Geometry: final body of the model. Coordinates: model frame, mm. Face numbers are marked on the shaded views. Give positions to 0.01 mm unless a question says otherwise; leave off trailing zeros. Loops run counter-clockwise (first coordinate to the right, second up) from the corner with the lowest first, then second, coordinate; pieces in that order, holes last.
1. Section B-B, the plane z = 1.15. Output: boundary loops of the cut face in (x, y).
2. Draft query along Y for the marked faces 1, 2 and 3. Return one class per face: +Y half, -Y half, draft (parallel to the pull), parting line (faces both ways), or undercut.
3. Section A-A, the plane y = 0. Output: boundary loops of the cut face in (x, z), then the cut area to 3 significant figures.
4. Material intervals for line 1 along Y through (x, z) = (0, 1.5); line 2 along Y through (x, z) = (-3.5, 2.55); line 3 along X through (y, z) = (-15.5, 2.9), sorted ascending.
5. First-contact query: P1, Ø1, axis at y = -17.5, z = 1, coming from the +X side; P2, Ø13, axis at x = 0, y = 0, coming from the +Z side; P3, Ø4, axis at x = 27, y = -12, coming from the +Z side; P4, Ø5.5, axis at x = 0, y = 14, coming from the +Z side. Flat tips, straight axial feed; report the tip coordinate or a pass-through.
6. Section C-C, the plane x = 14. Output: boundary loops of the cut face in (y, z).
from build123d import *

# Parameters (mm, degrees)
SKETCH1_R                                           = 36.8
BOSS_EXTRUDE1_DEPTH                                 = 5
CUT_EXTRUDE1_REACH                                  = 54.283
SKETCH2_R                                           = 4
CUT_EXTRUDE2_DEPTH                                  = 2
CUT_EXTRUDE3_DEPTH                                  = 2
CSK_FOR_M3_FLAT_COUNTERSUNK_HEAD_SCREW1_D           = 3.4
CSK_FOR_M3_FLAT_COUNTERSUNK_HEAD_SCREW1_DEPTH       = 9
CSK_FOR_M3_FLAT_COUNTERSUNK_HEAD_SCREW1_CSINK_D     = 6
CSK_FOR_M3_FLAT_COUNTERSUNK_HEAD_SCREW1_CSINK_ANGLE = 90
CSK_FOR_M3_FLAT_COUNTERSUNK_HEAD_SCREW1_TIP         = 1.021463052


with BuildPart() as part:
    # Sketch1 → Boss-Extrude1 (new body)
    with BuildSketch(Plane.XY):
        Circle(SKETCH1_R)
    extrude(amount=BOSS_EXTRUDE1_DEPTH)

    # Sketch2 → Cut-Extrude1 (cut, up to next)
    with BuildSketch(Plane.XY.offset(5), mode=Mode.PRIVATE) as cut_extrude1_sk1:
        Circle(SKETCH2_R)
    cut_extrude1_tool1 = extrude(cut_extrude1_sk1.sketch, amount=-CUT_EXTRUDE1_REACH, mode=Mode.PRIVATE) & part.part
    add(cut_extrude1_tool1.solids().sort_by_distance((0, 0, 5))[0], mode=Mode.SUBTRACT)

    # Sketch3 → Cut-Extrude2 (cut)
    with BuildSketch(Plane.XY.offset(5)):
        with BuildLine():
            ThreePointArc((24.47031025, -11.410693067), (25.75035767, -8.119056587), (26.589809331, -4.688500797))
            ThreePointArc((26.589809331, -4.688500797), (30.065177123, -2.255022071), (32.498655849, -5.730389863))
            ThreePointArc((32.498655849, -5.730389863), (31.472659375, -9.923291384), (29.908156972, -13.946402637))
            ThreePointArc((29.908156972, -13.946402637), (25.921378826, -15.397471213), (24.47031025, -11.410693067))
        make_face()
    extrude(amount=-CUT_EXTRUDE2_DEPTH, mode=Mode.SUBTRACT)

    # Sketch4 → Cut-Extrude3 (cut)
    with BuildSketch(Plane.XY.offset(5)):
        with BuildLine():
            ThreePointArc((-20.316828686, 26.004354869), (-23.537264822, 23.130005722), (-26.354971832, 19.859895764))
            ThreePointArc((-26.354971832, 19.859895764), (-25.764510371, 15.658544164), (-21.563158771, 16.249005625))
            ThreePointArc((-21.563158771, 16.249005625), (-19.257762127, 18.924550136), (-16.622859834, 21.276290347))
            ThreePointArc((-16.622859834, 21.276290347), (-16.105811999, 25.487307034), (-20.316828686, 26.004354869))
        make_face()
    extrude(amount=-CUT_EXTRUDE3_DEPTH, mode=Mode.SUBTRACT)

    # CSK for M3 Flat Countersunk Head Screw1
    with Locations(Plane.XY.offset(5)):
        with Locations((0, 14), (14, 0), (0, -14), (-14, 0)):
            CounterSinkHole(CSK_FOR_M3_FLAT_COUNTERSUNK_HEAD_SCREW1_D / 2, CSK_FOR_M3_FLAT_COUNTERSUNK_HEAD_SCREW1_CSINK_D / 2, depth=CSK_FOR_M3_FLAT_COUNTERSUNK_HEAD_SCREW1_DEPTH, counter_sink_angle=CSK_FOR_M3_FLAT_COUNTERSUNK_HEAD_SCREW1_CSINK_ANGLE)
            with Locations((0, 0, -(CSK_FOR_M3_FLAT_COUNTERSUNK_HEAD_SCREW1_DEPTH + CSK_FOR_M3_FLAT_COUNTERSUNK_HEAD_SCREW1_TIP / 2))):  # 118° drill point
                Cone(0, CSK_FOR_M3_FLAT_COUNTERSUNK_HEAD_SCREW1_D / 2, CSK_FOR_M3_FLAT_COUNTERSUNK_HEAD_SCREW1_TIP, mode=Mode.SUBTRACT)


solid = part.part
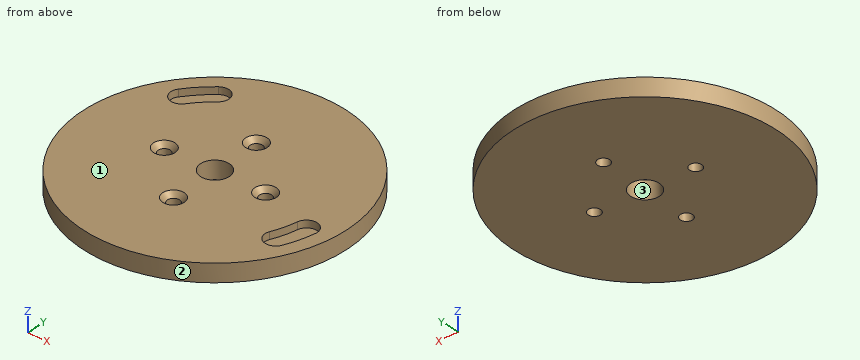
Answers below:
1. outline: circle Ø73.6 at (0, 0); hole circle Ø3.4 at (-14, 0); hole circle Ø8 at (0, 0); hole circle Ø3.4 at (0, -14); hole circle Ø3.4 at (0, 14); hole circle Ø3.4 at (14, 0)
2. face 1: draft
2. face 2: parting line
2. face 3: undercut
3. outline: (-36.8, 0) - (-15.7, 0) - (-15.7, 3.7) - (-17, 5) - (-36.8, 5) - close; (-12.3, 0) - (-4, 0) - (-4, 5) - (-11, 5) - (-12.3, 3.7) - close; (4, 0) - (12.3, 0) - (12.3, 3.7) - (11, 5) - (4, 5) - close; (15.7, 0) - (36.8, 0) - (36.8, 5) - (17, 5) - (15.7, 3.7) - close
3. area: 291 mm2
4. line 1: y = -36.8 to -15.7, -12.3 to -4, 4 to 12.3, 15.7 to 36.8
4. line 2: y = -36.63 to -1.94, 1.94 to 36.63
4. line 3: x = -33.38 to -0.8, 0.8 to 33.38
5. P1: stops at x = 32.64
5. P2: stops at z = 5
5. P3: stops at z = 3
5. P4: stops at z = 4.75
6. outline: (-34.03, 0) - (-1.7, 0) - (-1.7, 3.7) - (-3, 5) - (-34.03, 5) - close; (1.7, 0) - (34.03, 0) - (34.03, 5) - (3, 5) - (1.7, 3.7) - close
